Build history of the part. All positions in model axes, mm. A direction names the side the tool comes from. Coordinates: 2 decimals unless noted, no trailing zeros. Loops run counter-clockwise (first coordinate to the right, second up) from the corner with the lowest first, then second, coordinate; pieces in that order, holes last. Notation, with made-up numbers: (51.5, 43) - (66.5, 43) arc R14 cw to (66.5, 54) - close; hole circle Ø3 at (53.5, 73). An arc over 180 degrees is marked (long way). One line per item, written item: value.
Autodesk Inventor part; units mm, degrees
ref_plane "YZ Plane" through (0, 0, 0) normal (1, 0, 0) x (0, 1, 0)
ref_plane "XZ Plane" through (0, 0, 0) normal (0, 1, 0) x (-1, 0, 0)
ref_plane "XY Plane" through (0, 0, 0) normal (0, 0, 1) x (1, 0, 0)
sketch "Sketch1" plane through (0, 0, 0) normal (0, 1, 0) x (-1, 0, 0)
  line L0 (-50.5, 29.5) -> (50.5, 29.5)
  line L1 (50.5, 29.5) -> (50.5, -29.5)
  line L2 (50.5, -29.5) -> (-50.5, -29.5)
  line L3 (-50.5, -29.5) -> (-50.5, 29.5)
  line L4 (-50.5, 29.5) -> (50.5, -29.5) construction
  line L5 (50.5, 29.5) -> (-50.5, -29.5) construction
  line L6 (5.5, 16.6667) -> (10.5, 16.6667)
  line L7 (10.5, 6.6667) -> (5.5, 6.6667)
  line L8 (5.5, 6.6667) -> (5.5, 16.6667)
  line L9 (5.5, 16.6667) -> (10.5, 6.6667) construction
  line L10 (10.5, 16.6667) -> (5.5, 6.6667) construction
  line L11 (5.5, -16.6667) -> (10.5, -16.6667)
  line L12 (10.5, -6.6667) -> (5.5, -6.6667)
  line L13 (5.5, -16.6667) -> (10.5, -6.6667) construction
  line L14 (10.5, -16.6667) -> (5.5, -6.6667) construction
  line L15 (10.5, 10) -> (20.5, 10)
  line L16 (20.5, 11) -> (20.5, 9)
  line L17 (20.5, 9) -> (10.5, 9)
  line L18 (20.5, 11) -> (10.5, 11)
  line L19 (10.5, -10) -> (15.5, -10)
  line L20 (15.5, -9) -> (15.5, -11)
  line L21 (5.5, 10) -> (0.5, 10)
  line L22 (0.5, 11) -> (0.5, 9)
  line L23 (0.5, 11) -> (5.5, 11)
  line L24 (0.5, 9) -> (5.5, 9)
  line L25 (15.5, -11) -> (10.5, -11)
  line L26 (15.5, -9) -> (10.5, -9)
  line L27 (48.5, 27.5) -> (20.5, 27.5)
  line L28 (20.5, 27.5) -> (20.5, -27.5)
  line L29 (20.5, -27.5) -> (48.5, -27.5)
  line L30 (48.5, -27.5) -> (48.5, 27.5)
  line L31 (10.5, 16.6667) -> (10.5, 13.3333)
  line L32 (10.5, 13.3333) -> (10.5, 10)
  line L33 (10.5, 10) -> (10.5, 6.6667)
  line L34 (5.5, -16.6667) -> (5.5, -13.3333)
  line L35 (5.5, -13.3333) -> (5.5, -10)
  line L36 (5.5, -10) -> (5.5, -6.6667)
  line L37 (0.5, -11) -> (0.5, -9)
  line L38 (5.5, -10) -> (0.5, -10)
  line L39 (0.5, -11) -> (5.5, -11)
  line L40 (0.5, -9) -> (5.5, -9)
  line L41 (10.5, -16.6667) -> (10.5, -6.6667)
  line L42 (8, 11.6667) -> (8, -11.6667)
  line L43 (50.5, 0) -> (-50.5, 0)
  point P0 (0, 0)
  point P1 (0, 29.5)
  point P2 (0, -29.5)
  point P3 (8, 0)
  dimension "d0" = 101
  dimension "d1" = 59
  dimension "d4" = 5
  dimension "d5" = 10
  dimension "d6" = 10
  dimension "d7" = 2
  dimension "d8" = 5
  dimension "d14" = 20
  dimension "d15" = 2
  dimension "d16" = 2
  dimension "d17" = 55
  dimension "d18" = 2
  dimension "d19" = 28
  dimension "d27" = 42.5
extrude "Extrusion4" add sketch "Sketch1" along normal blind 2 contours L0 L1 L43 L30 L27 L28 L18 L32 L31 L6 L8 L23 L22 L24 L7 L42 L3 | L43 L28 L29 L30 L1 L2 L3 | L42 L7 L33 L17 L28 L43
properties part number "Lag2"
Item 1: Cut at B-B, the plane y = 1.6. Give the number of separate pieces and of enclosed holes in the cut face, then the cut area to 3 significant figures.
Check result:
separate pieces: 1
enclosed holes: 2
area: 4,270 mm^2
Item 2: Pull direction Z, two halves, no side cores. Call faces 1 (the face through (12, 2, 0)), 2 (the face through (-1, 1, -29.5)), 3 (the face through (-20.5, 1, 19)): released by +Z, released by -Z, zero draft, split by the parting line, or undercut.
Check result:
face 1: zero draft
face 2: released by -Z
face 3: undercut
Item 3: Cut at A-A, the plane x = -8. Write the cut outline in (y, z).
Check result:
outline: (0, -29.5) - (2, -29.5) - (2, -16.67) - (0, -16.67) - close; (0, -6.67) - (2, -6.67) - (2, 6.67) - (0, 6.67) - close; (0, 16.67) - (2, 16.67) - (2, 29.5) - (0, 29.5) - close
Item 4: Probe probe 1 along X at (y, z) = (1.25, -13.5); probe 2 along Z at (x, y) = (-4, 1); probe 3 along X at (y, z) = (1.1, -3.5). List the from-to ranges inside material, lowest first. Write a range as from..to.
Check result:
probe 1: x = -50.5..-48.5, -20.5..-10.5, -5.5..50.5
probe 2: z = -29.5..-11, -9..9, 11..29.5
probe 3: x = -50.5..-48.5, -20.5..50.5
Item 5: Cut at C-C, the plane z = 1.5. Write the cut outline in (x, y), then the cut area to 3 significant figures.
Check result:
outline: (-50.5, 0) - (-48.5, 0) - (-48.5, 2) - (-50.5, 2) - close; (-20.5, 0) - (50.5, 0) - (50.5, 2) - (-20.5, 2) - close
area: 146 mm^2
Item 6: Tool access for faces 4 (the face through (12, 0, 0)), 5 (the face through (-48.5, 1, 0)): list every direction of +Z, -Z, +X, -X, +Y, -Y with a clear straight run to the whole face (end or side of a thin tool).
Check result:
face 4: +Z, -Z, +X, -X, -Y
face 5: +Y, -Y
